Here's how the part is built. I have some questions about the finished solid (model axes, mm). A direction names the side the tool comes from. Round coordinates to 2 decimals unless told otherwise and drop trailing zeros. Loops run counter-clockwise (first coordinate to the right, second up) from the corner with the lowest first, then second, coordinate; pieces in that order, holes last. Notation, with made-up numbers: M 84,53.5 L 88,53.5 A26 ccw 88,82.5 Z; hole C 8.5,0.5 d7. An arc over 180 degrees is marked long. Use a Markdown table: item, result.
from build123d import *

# Parameters (mm, degrees)
F0_R          = 4
F1_DEPTH      = 42.5
F1_DEPTH_BACK = 42.5
F2_W          = 8
F2_H          = 8
F3_DEPTH      = 25
F4_W          = 3.5
F4_H          = 8
F5_DEPTH      = 70
F6_R          = 2
F7_DEPTH      = 25
F8_R          = 2
F9_DEPTH      = 25
F10_R         = 3.99999
F11_R         = 2.1
F12_DEPTH     = 82.3766380975
F14_DEPTH     = 16


# Not quite as in the source:
# - a fillet or chamfer is up to 0.001 mm smaller than in the source, because OpenCascade refuses the exact size


with BuildPart() as f1:
    # F0 (on Right) → F1 (new body, two sides)
    with BuildSketch(Plane.YZ) as f1_sk:
        Circle(F0_R)
    extrude(amount=F1_DEPTH)
    extrude(f1_sk.sketch, amount=-F1_DEPTH_BACK)

    # F2 (on Top) → F3 (cut)
    with BuildSketch(Plane.XY):
        with Locations((-4, 0)):
            Rectangle(F2_W, F2_H)
        with Locations((4, 0)):
            Rectangle(F2_W, F2_H)
    extrude(amount=F3_DEPTH, mode=Mode.SUBTRACT)

    # F4 (on Front) → F5 (join)
    with BuildSketch(Plane.XZ):
        with Locations((38.1256380975, 0)):
            Rectangle(F4_W, F4_H)
        with Locations((-38.1256380975, 0)):
            Rectangle(F4_W, F4_H)
    extrude(amount=-F5_DEPTH)

    # F6 (on face) → F7 (cut)
    with BuildSketch(Plane.YZ.offset(42.5)):
        Circle(F6_R)
    extrude(amount=-F7_DEPTH, mode=Mode.SUBTRACT)

    # F8 (on face) → F9 (cut)
    with BuildSketch(Plane(origin=(-42.5, 0, 0), x_dir=(0, -1, 0), z_dir=(-1, 0, 0))):
        Circle(F8_R)
    extrude(amount=-F9_DEPTH, mode=Mode.SUBTRACT)

    # F10 (radius 4 in the source; OpenCascade refuses exactly that, so slightly less here)
    f10_edges = [f1.edges().sort_by_distance(p)[0] for p in [
        (38.125638, 70, 4),
        (38.125638, 70, -4),
        (-38.125638, 70, 4),
        (-38.125638, 70, -4),
    ]]
    fillet(f10_edges, radius=F10_R)

    # F11 (on face) → F12 (cut, through all)
    with BuildSketch(Plane(origin=(-39.8756380975, 0, 0), x_dir=(0, -1, 0), z_dir=(-1, 0, 0))):
        with Locations((-66, 0)):
            Circle(F11_R)
        with Locations((-33.5, 0)):
            Circle(F11_R)
    extrude(amount=-F12_DEPTH, mode=Mode.SUBTRACT)

    # F13 (on face) → F14 (join, through all)
    with BuildSketch(Plane(origin=(8, 0, 0), x_dir=(0, -1, 0), z_dir=(-1, 0, 0))):
        with BuildLine():
            ThreePointArc((-3.848557921, 1.0902302184), (-3.9619585866, 0.5503491238), (-4, 0))
            Line((-4, 0), (4, 0))
            ThreePointArc((4, 0), (3.9619585866, 0.5503491238), (3.848557921, 1.0902302184))
            Line((3.848557921, 1.0902302184), (-3.848557921, 1.0902302184))
        make_face()
    extrude(amount=F14_DEPTH)


solid = f1.part
1. We'd pull the mould along Y, two halves only. Please class faces 4 (the face through (-38.101, 68.797, -2.859)), 5 (the face through (-38, 33, 4)), 6 (the face through (38.1, 35.6, 0.09)): +Y half, -Y half, draft (parallel to the pull), parting line (faces both ways), or undercut.
Answer sheet:
| item | result |
|---|---|
| face 4 | +Y half |
| face 5 | draft |
| face 6 | undercut |
2. Imagine slicing it at C-C, the plane x = 26. Write out the boundary of the cut face in (y, z).
Answer sheet:
| item | result |
|---|---|
| outline | C 0,0 d8; hole C 0,0 d4 |
3. Imagine slicing it at B-B, the plane y = 20.5. Write out the boundary of the cut face in (x, z).
Answer sheet:
| item | result |
|---|---|
| outline | M -39.88,-4 L -36.38,-4 L -36.38,4 L -39.88,4 Z; M 36.38,-4 L 39.88,-4 L 39.88,4 L 36.38,4 Z |
4. Imagine slicing it at A-A, the plane y = 33.5. Write out the boundary of the cut face in (x, z).
Answer sheet:
| item | result |
|---|---|
| outline | M -39.88,-4 L -36.38,-4 L -36.38,-2.1 L -39.88,-2.1 Z; M -39.88,2.1 L -36.38,2.1 L -36.38,4 L -39.88,4 Z; M 36.38,-4 L 39.88,-4 L 39.88,-2.1 L 36.38,-2.1 Z; M 36.38,2.1 L 39.88,2.1 L 39.88,4 L 36.38,4 Z |
5. For pin 1 Ø4 at (y, z) = (42.5, -1.5) entering from -X; pin 2 Ø3.5 at (y, z) = (0, 0) entering from -X; pin 3 Ø3.5 at (y, z) = (33.5, 0) entering from +X; pin 4 Ø3 at (x, z) = (29.5, -2) entering from -Y, each with a flat end and sliding along its axis, tell me the tip position at first contact or that it passes through.
Answer sheet:
| item | result |
|---|---|
| pin 1 | x = -39.88 |
| pin 2 | x = -17.5 |
| pin 3 | through |
| pin 4 | y = -3.97 |
6. I need wall thicknesses on probe 1 along X at (y, z) = (35, 2.5); probe 2 along Z at (x, y) = (-24, 0); probe 3 along Z at (x, y) = (-37.8, 66). Which ranges of each line are inside material? Lowest first, please. Write a range as from..to.
Answer sheet:
| item | result |
|---|---|
| probe 1 | -39.88..-36.38, 36.38..39.88 |
| probe 2 | -4..-2, 2..4 |
| probe 3 | -4..-2.1, 2.1..4 |
7. Which directions (+Z, -Z, +X, -X, +Y, -Y) give clear straight access to the entire face, cutting with the end or side of a thin tool? Please do faces 1 (the face through (8, 0, 2)), 2 (the face through (30, 0, -2)), 3 (the face through (-30, 0, -2)).
Answer sheet:
| item | result |
|---|---|
| face 1 | +Z, +Y, -Y |
| face 2 | +X |
| face 3 | -X |
8. Imagine slicing it at D-D, the plane x = -6.5. Write out the boundary of the cut face in (y, z), then the cut area to 3 significant figures.
Answer sheet:
| item | result |
|---|---|
| outline | M -3.85,1.09 A4 ccw long 3.85,1.09 Z |
| area | 33.7 mm2 |
